Can you work these out from the model? Positions are in its coordinate system, mm. Round coordinates to 2 decimals unless told otherwise and drop trailing zeros. Order: outer loops, then holes, each group sorted by start corner. A loop starts at its lowest first (then second) coordinate and runs counter-clockwise, first axis right, second up.
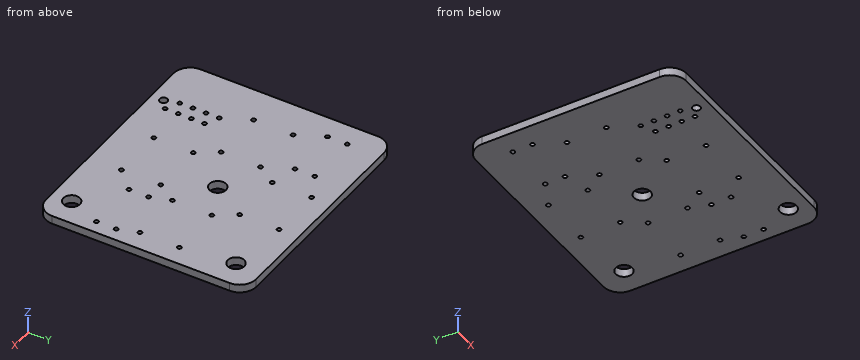
Autodesk Inventor part; units mm, degrees
ref_plane "Plan YZ" through (0, 0, 0) normal (1, 0, 0) x (0, 1, 0)
ref_plane "Plan XZ" through (0, 0, 0) normal (0, 1, 0) x (-1, 0, 0)
ref_plane "Plan XY" through (0, 0, 0) normal (0, 0, 1) x (1, 0, 0)
sketch "Esquisse1" plane through (0, 0, 0) normal (0, 0, 1) x (1, 0, 0)
  point P0 (0, 0)
sketch "Esquisse6" plane through (0, 0, 0) normal (0, 0, 1) x (1, 0, 0)
  arc A0 (135.89, -68.58) -> (132.715, -71.755) centre (135.89, -71.755) ccw
  line L0 (132.715, -71.755) -> (132.715, -106.045)
  arc A1 (132.715, -106.045) -> (135.89, -109.22) centre (135.89, -106.045) ccw
  line L1 (135.89, -109.22) -> (175.895, -109.22)
  arc A2 (175.895, -109.22) -> (179.07, -106.045) centre (175.895, -106.045) ccw
  line L2 (179.07, -106.045) -> (179.07, -71.755)
  arc A3 (179.07, -71.755) -> (175.895, -68.58) centre (175.895, -71.755) ccw
  line L3 (175.895, -68.58) -> (135.89, -68.58)
  circle A4 centre (142.24, -96.52) radius 0.4
  circle A5 centre (144.78, -97.79) radius 0.4
  circle A6 centre (142.24, -99.06) radius 0.4
  circle A7 centre (144.78, -100.33) radius 0.4
  circle A8 centre (142.24, -101.6) radius 0.4
  circle A9 centre (144.78, -102.87) radius 0.4
  circle A10 centre (142.24, -104.14) radius 0.4
  circle A11 centre (144.78, -105.41) radius 0.4
  circle A12 centre (137.16, -78.74) radius 0.4
  circle A13 centre (147.32, -78.74) radius 0.4
  circle A14 centre (166.37, -99.06) radius 0.4
  circle A15 centre (176.53, -99.06) radius 0.4
  circle A16 centre (176.53, -95.25) radius 0.4
  circle A17 centre (166.37, -95.25) radius 0.4
  circle A18 centre (147.32, -74.93) radius 0.4
  circle A19 centre (137.16, -74.93) radius 0.4
  circle A20 centre (149.86, -83.82) radius 0.4
  circle A21 centre (139.7, -83.82) radius 0.4
  circle A22 centre (149.86, -91.44) radius 0.4
  circle A23 centre (139.7, -91.44) radius 0.4
  circle A24 centre (162.56, -95.25) radius 0.4
  circle A25 centre (152.4, -95.25) radius 0.4
  circle A26 centre (162.56, -102.87) radius 0.4
  circle A27 centre (152.4, -102.87) radius 0.4
  circle A28 centre (175.26, -83.82) radius 0.4
  circle A29 centre (165.1, -83.82) radius 0.4
  circle A30 centre (175.26, -91.44) radius 0.4
  circle A31 centre (165.1, -91.44) radius 0.4
  circle A32 centre (162.56, -72.39) radius 0.4
  circle A33 centre (152.4, -72.39) radius 0.4
  circle A34 centre (162.56, -80.01) radius 0.4
  circle A35 centre (152.4, -80.01) radius 0.4
  circle A36 centre (142.98, -106.81) radius 0.75
  circle A37 centre (158.115, -86.995) radius 1.6
  circle A38 centre (173.99, -105.41) radius 1.6
  circle A39 centre (173.99, -73.66) radius 1.6
extrude "manette_2019_boutons.kicad_pcb_Contour" add sketch "Esquisse6" along normal blind 1.6
properties part number "manette_2019_boutons.kicad_pcb_Contour" material "."
(1) I want a section at A-A, the plane x = 157.5. List the corners of the cut face in (y, z) for me.
(2) Please list where these lines run through material, in increasing order: probe 1 along Y at (x, z) = (152.4, 0.5); probe 2 along X at (y, z) = (-80.01, 1.1) (3 decimals); probe 3 along Y at (x, z) = (137.16, 0.55).
(3) I want a section at B-B, the plane y = -86. List the corners of the cut face in (x, z) for me (3 decimals), plus the area to 3 significant figures.
(4) I want a section at D-D, the plane z = 0.8. Give the number of separate pieces and of enclosed holes in the cut face, plus the area to 3 significant figures.
(5) I want a section at C-C, the plane x = 173. List the corners of the cut face in (y, z) for me, plus the area to 3 significant figures.
Ans:
1. outline: (-109.22, 0) - (-88.47, 0) - (-88.47, 1.6) - (-109.22, 1.6) - close; (-85.52, 0) - (-68.58, 0) - (-68.58, 1.6) - (-85.52, 1.6) - close
2. probe 1: y = -109.22 to -103.27, -102.47 to -95.65, -94.85 to -80.41, -79.61 to -72.79, -71.99 to -68.58
2. probe 2: x = 132.715 to 152, 152.8 to 162.16, 162.96 to 179.07
2. probe 3: y = -109.22 to -79.14, -78.34 to -75.33, -74.53 to -68.58
3. outline: (132.715, 0) - (156.862, 0) - (156.862, 1.6) - (132.715, 1.6) - close; (159.368, 0) - (179.07, 0) - (179.07, 1.6) - (159.368, 1.6) - close
3. area: 70.2 mm2
4. separate pieces: 1
4. enclosed holes: 36
4. area: 1,830 mm2
5. outline: (-109.22, 0) - (-106.67, 0) - (-106.67, 1.6) - (-109.22, 1.6) - close; (-104.15, 0) - (-74.92, 0) - (-74.92, 1.6) - (-104.15, 1.6) - close; (-72.4, 0) - (-68.58, 0) - (-68.58, 1.6) - (-72.4, 1.6) - close
5. area: 57.0 mm2
